Source: CAD feature listing. Evaluate the final solid. Frame: model axes, mm. A direction names the side the tool comes from. Give positions to 0.01 mm unless a question says otherwise; leave off trailing zeros. Order: outer loops, then holes, each group sorted by start corner. A loop starts at its lowest first (then second) coordinate and runs counter-clockwise, first axis right, second up. Notation, with made-up numbers: (63, -9.5) - (85, -9.5) arc R24 cw to (85, 3.5) - close; hole circle Ø6 at (49.25, -8.75). An arc over 180 degrees is marked (long way). Use CSV: the item, a comma, the result in double quotes.
```python
from build123d import *

# Parameters (mm, degrees)
EXTRUDE_1_DEPTH          = 230
EXTRUDE_2_DEPTH          = 90
EXTRUDE_3_DEPTH          = 90
EXTRUDE_3_DEPTH_BACK     = 145
SKETCH_5_W               = 200
SKETCH_5_H               = 220
SKETCH_4_R               = 120
CUT_EXTRUDE_1_DEPTH      = 745.865759718
CUT_EXTRUDE_2_REACH      = 590.605
CUT_EXTRUDE_2_END_RADIUS = 120
SKETCH_6_R               = 90
CUT_EXTRUDE_3_REACH      = 626.355
SKETCH_7_R               = 10
SKETCH_8_R               = 5
CUT_EXTRUDE_4_DEPTH      = 30
FILLET_1_R               = 10
FILLET_2_R               = 10


with BuildPart() as part:
    # Эскиз1 → Бобышка-Вытянуть1 (new body)
    with BuildSketch(Plane.XY):
        Polygon((-50, -200), (-50, -138.564064606), (-145, -83.715789032), (-145, 83.715789032), (0, 167.431578065), (145, 83.715789032), (145, -83.715789032), (50, -138.564064606), (50, -200), (135, -200), (135, -300), (-135, -300), (-135, -200), align=None)
    extrude(amount=EXTRUDE_1_DEPTH)

    # Эскиз2 → Бобышка-Вытянуть2 (add)
    with BuildSketch(Plane.XY.offset(230)):
        Polygon((0, 181.865334795), (-157.5, 90.932667397), (-157.5, -90.932667397), (0, -181.865334795), (157.5, -90.932667397), (157.5, 90.932667397), align=None)
    extrude(amount=EXTRUDE_2_DEPTH)

    # Зеркальное отражение1: part across plane


with BuildPart() as part_1:
    add(part.part)
    add(part.part.mirror(Plane.XY))

    # Эскиз5 → Бобышка-Вытянуть3 (add, two sides: drawn at the far end of the back side and taken through both)
    with BuildSketch(Plane(origin=(145, 0, 0), x_dir=(0, 0, -1), z_dir=(1, 0, 0)).offset(-EXTRUDE_3_DEPTH_BACK)):
        with Locations((90, 0)):
            Rectangle(SKETCH_5_W, SKETCH_5_H)
    extrude(amount=EXTRUDE_3_DEPTH + EXTRUDE_3_DEPTH_BACK)

    # Эскиз4 → Вырез-Вытянуть1 (cut, through all)
    with BuildSketch(Plane.XY.offset(320)):
        Circle(SKETCH_4_R)
    extrude(amount=-CUT_EXTRUDE_1_DEPTH, mode=Mode.SUBTRACT)

    # Вырез-Вытянуть2: up to this cylinder (the profile starts outside it)
    cut_extrude_2_end = Plane(origin=(0, 0, -90), z_dir=(0, 0, 1)) * Cylinder(CUT_EXTRUDE_2_END_RADIUS, 1422.21, mode=Mode.PRIVATE)
    # Эскиз6 → Вырез-Вытянуть2 (cut, up to the surface)
    with BuildSketch(Plane(origin=(235, 0, 0), x_dir=(0, 0, -1), z_dir=(1, 0, 0)), mode=Mode.PRIVATE) as cut_extrude_2_sk1:
        with Locations((90, 5)):
            Circle(SKETCH_6_R)
    cut_extrude_2_tool1 = extrude(cut_extrude_2_sk1.sketch, amount=-CUT_EXTRUDE_2_REACH, mode=Mode.PRIVATE) - cut_extrude_2_end
    add(cut_extrude_2_tool1.solids().sort_by_distance((235, 5, -90))[0], mode=Mode.SUBTRACT)

    # Эскиз7 → Вырез-Вытянуть3 (cut, up to next)
    with BuildSketch(Plane.XZ.offset(300), mode=Mode.PRIVATE) as cut_extrude_3_sk1:
        with Locations(Location((115, 210, 0), (0, 0, 270))):
            Circle(SKETCH_7_R)
    cut_extrude_3_tool1 = extrude(cut_extrude_3_sk1.sketch, amount=-CUT_EXTRUDE_3_REACH, mode=Mode.PRIVATE) & part_1.part
    # Эскиз7 → Вырез-Вытянуть3 (cut, up to next)
    with BuildSketch(Plane.XZ.offset(300), mode=Mode.PRIVATE) as cut_extrude_3_sk2:
        with Locations(Location((-115, 210, 0), (0, 0, 270))):
            Circle(SKETCH_7_R)
    cut_extrude_3_tool2 = extrude(cut_extrude_3_sk2.sketch, amount=-CUT_EXTRUDE_3_REACH, mode=Mode.PRIVATE) & part_1.part
    # Эскиз7 → Вырез-Вытянуть3 (cut, up to next)
    with BuildSketch(Plane.XZ.offset(300), mode=Mode.PRIVATE) as cut_extrude_3_sk3:
        with Locations(Location((115, -210, 0), (0, 0, 270))):
            Circle(SKETCH_7_R)
    cut_extrude_3_tool3 = extrude(cut_extrude_3_sk3.sketch, amount=-CUT_EXTRUDE_3_REACH, mode=Mode.PRIVATE) & part_1.part
    # Эскиз7 → Вырез-Вытянуть3 (cut, up to next)
    with BuildSketch(Plane.XZ.offset(300), mode=Mode.PRIVATE) as cut_extrude_3_sk4:
        with Locations(Location((-115, -210, 0), (0, 0, 270))):
            Circle(SKETCH_7_R)
    cut_extrude_3_tool4 = extrude(cut_extrude_3_sk4.sketch, amount=-CUT_EXTRUDE_3_REACH, mode=Mode.PRIVATE) & part_1.part
    add(cut_extrude_3_tool1.solids().sort_by_distance((115, -300, 210))[0], mode=Mode.SUBTRACT)
    add(cut_extrude_3_tool2.solids().sort_by_distance((-115, -300, 210))[0], mode=Mode.SUBTRACT)
    add(cut_extrude_3_tool3.solids().sort_by_distance((115, -300, -210))[0], mode=Mode.SUBTRACT)
    add(cut_extrude_3_tool4.solids().sort_by_distance((-115, -300, -210))[0], mode=Mode.SUBTRACT)

    # Эскиз8 → Вырез-Вытянуть4 (cut)
    with BuildSketch(Plane(origin=(235, 0, 0), x_dir=(0, 0, -1), z_dir=(1, 0, 0))):
        with Locations((0, 100)):
            Circle(SKETCH_8_R)
        with Locations((0, -100)):
            Circle(SKETCH_8_R)
        with Locations((180, 100)):
            Circle(SKETCH_8_R)
        with Locations((180, -100)):
            Circle(SKETCH_8_R)
    extrude(amount=-CUT_EXTRUDE_4_DEPTH, mode=Mode.SUBTRACT)

    # Скругление1
    fillet_1_edges = [part_1.edges().sort_by_distance(p)[0] for p in [
        (-135, -250, 230),
        (135, -250, 230),
        (-135, -250, -230),
        (135, -250, -230),
    ]]
    fillet(fillet_1_edges, radius=FILLET_1_R)

    # Скругление2
    fillet_2_edges = [part_1.edges().sort_by_distance(p)[0] for p in [
        (167.237205584, 110, 10),
        (167.237205584, -110, -190),
        (167.237205584, 110, -190),
        (167.237205584, -110, 10),
    ]]
    fillet(fillet_2_edges, radius=FILLET_2_R)


solid = part_1.part
```
Item 1: Section C-C on y = -63. Return the cut outline in (x, z).
Filled in:
outline,"(-157.5, -320) - (-102.13, -320) - (-102.13, 320) - (-157.5, 320) - (-157.5, 230) - (-145, 230) - (-145, -230) - (-157.5, -230) - close; (102.13, -320) - (157.5, -320) - (157.5, -230) - (145, -230) - (145, -190) - (235, -190) - (235, -148.96) - (102.13, -148.96) - close; (102.13, -31.04) - (235, -31.04) - (235, 10) - (145, 10) - (145, 230) - (157.5, 230) - (157.5, 320) - (102.13, 320) - close"
Item 2: Mould query, pull axis Y, two halves, no side actions, for faces 1 (the flat face through (55.374, 135.461, 3.22)), 2 (the flat face through (2, -242, 230)), 3 (the flat face through (166, -110, -89)). Classes: released by +Y, released by -Y, zero draft, split by the parting line, or undercut.
Filled in:
face 1,"released by +Y"
face 2,"zero draft"
face 3,"undercut"
Item 3: Section A-A on z = -210. Return the cut outline in (x, y).
Filled in:
outline,"(-145, -83.72) - (-50, -138.56) - (-50, -200) - (-105, -200) - (-105, -300) - (105, -300) - (105, -200) - (50, -200) - (50, -138.56) - (145, -83.72) - (145, 83.72) - (0, 167.43) - (-145, 83.72) - close; (-135, -300) - (-125, -300) - (-125, -200) - (-135, -200) - close; (125, -300) - (135, -300) - (135, -200) - (125, -200) - close; hole circle Ø240 at (0, 0)"
Item 4: Material intervals for line 1 (Y direction, x = 132, z = -90); line 2 (X direction, y = -241, z = 210); line 3 (Y direction, x = 119.5, z = -41.5), sorted ascending. Write a range as from..to.
Filled in:
line 1,"y = -300..-200, -110..-85, 95..110"
line 2,"x = -135..-125, -105..105, 125..135"
line 3,"y = -300..-200, -110..-70.81, 80.81..110"
Item 5: First-contact query: pin 1 (3 mm diameter, centred on x = 84.5, z = -120.5, fed in from +Y); pin 2 (8 mm diameter, centred on y = -131, z = -68, fed in from +X); pin 3 (3 mm diameter, centred on x = -77.5, z = 196.5, fed in from +Y). Flat tips, straight axial feed; report the tip coordinate or a pass-through.
Filled in:
pin 1,"stops at y = 119.51"
pin 2,"stops at x = 70.03"
pin 3,"stops at y = 123.55"
Item 6: Set-up query: faces 4 (the flat face through (77.648, -137.036, -274.37)), 5 (the flat face through (145, 1, 122)), 6 (the flat face through (-71, 127, 230)). Return all of +Z, -Z, +X, -X, +Y, -Y with unobstructed straight access to the full face (end or side cutting, diameter ignored); none if empty.
Filled in:
face 4,"-Z, +X, -Y"
face 5,"+X, +Y, -Y"
face 6,"none"
Item 7: Section B-B on x = 181.5. Return the cut outline in (y, z).
Filled in:
outline,"(-110, -180) arc R10 ccw to (-100, -190) - (100, -190) arc R10 ccw to (110, -180) - (110, 0) arc R10 ccw to (100, 10) - (-100, 10) arc R10 ccw to (-110, 0) - close; hole circle Ø180 at (5, -90)"
Item 8: Section D-D on x = 38. Return the cut outline in (y, z), then the cut area to 3 significant figures.
Filled in:
outline,"(-300, -230) - (-159.93, -230) - (-159.93, -320) - (-113.82, -320) - (-113.82, 320) - (-159.93, 320) - (-159.93, 230) - (-300, 230) - close; (113.82, -320) - (159.93, -320) - (159.93, -230) - (145.49, -230) - (145.49, 230) - (159.93, 230) - (159.93, 320) - (113.82, 320) - close"
area,"117,000 mm2"
